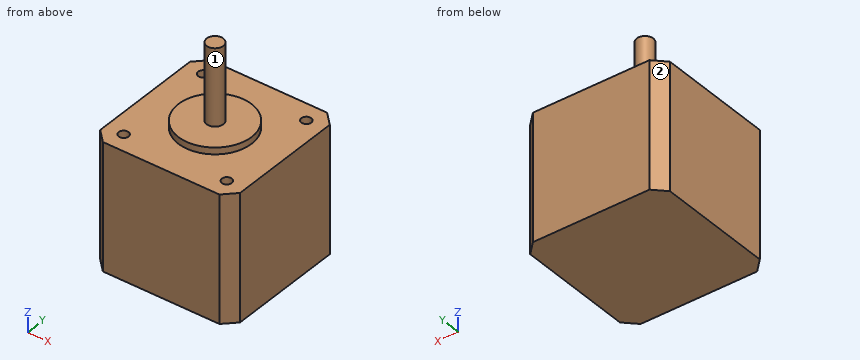
Autodesk Inventor part; units mm, degrees
ref_plane "YZ Plane" through (0, 0, 0) normal (1, 0, 0) x (0, 1, 0)
ref_plane "XZ Plane" through (0, 0, 0) normal (0, 1, 0) x (-1, 0, 0)
ref_plane "XY Plane" through (0, 0, 0) normal (0, 0, 1) x (1, 0, 0)
sketch "Sketch1" plane through (0, 0, 0) normal (0, 0, 1) x (1, 0, 0)
  line L0 (21, -21) -> (-21, -21)
  line L1 (-21, -21) -> (-21, 21)
  line L2 (-21, 21) -> (21, 21)
  line L3 (21, 21) -> (21, -21)
  line L4 (21, -21) -> (-21, 21) construction
  line L5 (-21, -21) -> (21, 21) construction
  point P0 (0, 0)
  dimension "d0" = 42
extrude "Extrusion1" add sketch "Sketch1" along normal blind 38
sketch "Sketch2" plane through (0, 0, 38) normal (0, 0, 1) x (1, 0, 0)
  point P0 (0, 0)
  point P1 (-15.5, 15.5)
  point P2 (-15.5, -15.5)
  point P3 (15.5, -15.5)
  point P4 (15.5, 15.5)
  dimension "d3" = 31
  dimension "d4" = 31
  dimension "d5" = 15.5
  dimension "d6" = 15.5
hole "Hole1" at (-15.5, 15.5, 38) at (-15.5, -15.5, 38) at (15.5, -15.5, 38) at (15.5, 15.5, 38) direction (0, 0, -1) diameter 3 depth 8 tip angle 118
chamfer "Chamfer1" distance 3.5 angle 45 4 edges at (21, 21, 19) (21, -21, 19) (-21, 21, 19) (-21, -21, 19)
sketch "Sketch3" plane through (0, 0, 38) normal (0, 0, 1) x (1, 0, 0)
  circle A0 centre (0, 0) radius 11
  dimension "d17" = 22
extrude "Extrusion2" add sketch "Sketch3" along normal blind 2
sketch "Sketch4" plane through (0, 0, 40) normal (0, 0, 1) x (1, 0, 0)
  circle A0 centre (0, 0) radius 11
  circle A1 centre (0, 0) radius 2.5
  dimension "d20" = 5
extrude "Extrusion3" add sketch "Sketch4" along normal blind 23 contours A1
properties part number "Z Axis Motor (Stepper)" material "Steel, Alloy"
Geometry check sheet. Reference: the model listing, model coordinates, mm. Face numbers are marked on the shaded views. A direction names the side the tool comes from. Coordinates: 2 decimals unless noted, no trailing zeros. Write each loop counter-clockwise with the first axis right and the second up, starting at its lowest first coordinate (ties: lowest second). Pieces come first, ordered by that corner, then holes. Notation, with made-up numbers: (81.5, 18.5) -> (91.5, 18.5) arc R21 cw to (91.5, 48.5) -> close; hole circle Ø11 at (2, 6.5). An arc over 180 degrees is marked (long way). One line per question, with ' | ' between items.
1. Cross-section at C-C on y = 10. Record the cut outline in (x, z).
Answers:
outline: (-21, 0) -> (21, 0) -> (21, 38) -> (4.58, 38) -> (4.58, 40) -> (-4.58, 40) -> (-4.58, 38) -> (-21, 38) -> close
2. Thickness scan on probe 1 along X at (y, z) = (15.5, 36); probe 2 along X at (y, z) = (15, 32); probe 3 along Z at (x, y) = (-13.5, 16.5). Record the ranges inside material, lowest first. Write a range as from..to.
Answers:
probe 1: x = -21..-17, -14..14, 17..21 | probe 2: x = -21..-16.91, -14.09..14.09, 16.91..21 | probe 3: z = 0..38
3. Set-up check for the marked faces 1 and 2: record each of +Z, -Z, +X, -X, +Y, -Y from which the full face is reachable in a straight line by a thin tool's end or side.
Answers:
face 1: +Z | face 2: +Z, -Z, -X, +Y
4. Cross-section at A-A on y = 0. Record the cut outline in (x, z).
Answers:
outline: (-21, 0) -> (21, 0) -> (21, 38) -> (11, 38) -> (11, 40) -> (2.5, 40) -> (2.5, 63) -> (-2.5, 63) -> (-2.5, 40) -> (-11, 40) -> (-11, 38) -> (-21, 38) -> close
5. Depth check by flat-ended pin: pin 1 Ø5 at (x, y) = (15.5, 15.5) entering from +Z; pin 2 Ø2 at (y, z) = (0.5, 51) entering from -X. Enter the tip coordinate at first touch or a pass-through.
Answers:
pin 1: stops at z = 38 | pin 2: stops at x = -2.5
6. Cross-section at B-B on x = -3.5. Record the cut outline in (y, z), and give its area (3 significant figures).
Answers:
outline: (-21, 0) -> (21, 0) -> (21, 38) -> (10.43, 38) -> (10.43, 40) -> (-10.43, 40) -> (-10.43, 38) -> (-21, 38) -> close | area: 1,640 mm²
